Geometry: final body of the model. Coordinates: model frame, mm. Face numbers are marked on the shaded views. A direction names the side the tool comes from. Give positions to 0.01 mm unless a question says otherwise; leave off trailing zeros. Write each loop counter-clockwise with the first axis right and the second up, starting at its lowest first coordinate (ties: lowest second). Pieces come first, ordered by that corner, then holes. Notation, with made-up numbers: M -30,79 L -2,79 A15 cw -2,96 Z; hole C 11,38 d3. An arc over 180 degrees is marked long. Answer as a JSON object with one key per item and string values.
Autodesk Inventor part; units mm, degrees
ref_plane "YZ Plane" through (0, 0, 0) normal (1, 0, 0) x (0, 1, 0)
ref_plane "XZ Plane" through (0, 0, 0) normal (0, 1, 0) x (-1, 0, 0)
ref_plane "XY Plane" through (0, 0, 0) normal (0, 0, 1) x (1, 0, 0)
sketch "スケッチ1" plane through (0, 0, 0) normal (0, 0, 1) x (1, 0, 0)
  line L0 (40.6372, 0) -> (-44.8968, 0)
  line L1 (0, -28.7297) -> (0, 26.7749)
  line L2 (17.5, -15) -> (-17.5, -15)
  line L3 (-17.5, -15) -> (-17.5, 15)
  line L4 (-17.5, 15) -> (17.5, 15)
  line L5 (17.5, 15) -> (17.5, -15)
  point P0 (0, 0)
  dimension "d0" = 35
  dimension "d1" = 30
extrude "押し出し1" add sketch "スケッチ1" along normal blind 30
sketch "スケッチ4" plane through (17.5, -15, 0) normal (1, 0, 0) x (0, 0, -1)
  line L0 (0, 30) -> (0, 0)
  line L1 (0, 30) -> (-30, 30)
  line L2 (-30, 0) -> (-30, 30)
  line L3 (0, 0) -> (-30, 0)
  line L4 (-30, 15) -> (0, 15)
  line L5 (0, 30) -> (-30, 30)
  line L6 (-15, 30) -> (-15, 0)
  circle A0 centre (-15, 15) radius 5
  dimension "d4" = 10
extrude "押し出し2" cut sketch "スケッチ4" against normal through all contours A0 L6 L4 | L4 L6 A0 | L6 L4 A0 | L6 A0 L4
sketch "スケッチ5" plane through (0, 0, 30) normal (0, 0, 1) x (1, 0, 0)
  line L0 (-5.9, -2.4) -> (-5.9, 2.4)
  line L1 (-2.4, -2.4) -> (-5.9, -2.4)
  line L2 (-2.4, -9) -> (-2.4, -2.4)
  line L3 (2.4, -9) -> (-2.4, -9)
  line L4 (2.4, -2.4) -> (2.4, -9)
  line L5 (5.9, -2.4) -> (2.4, -2.4)
  line L6 (5.9, 2.4) -> (5.9, -2.4)
  line L7 (2.4, 2.4) -> (5.9, 2.4)
  line L8 (2.4, 9) -> (2.4, 2.4)
  line L9 (-2.4, 9) -> (2.4, 9)
  line L10 (-2.4, 2.4) -> (-2.4, 9)
  line L11 (-5.9, 2.4) -> (-2.4, 2.4)
  ellipse E0 centre (0.5, 0) end of major axis (4.0355, 0) minor radius 2.5 (0, -2.4749) -> (0, 2.4749) ccw
  ellipse E1 centre (-0.5, 0) end of major axis (-4.0355, 0) minor radius 2.5 (0, 2.4749) -> (0, -2.4749) ccw
  line L12 (-2.6, 9.2) -> (2.6, 9.2)
  line L13 (2.6, 9.2) -> (2.6, 2.6)
  line L14 (2.6, 2.6) -> (6.1, 2.6)
  line L15 (6.1, 2.6) -> (6.1, -2.6)
  line L16 (6.1, -2.6) -> (2.6, -2.6)
  line L17 (2.6, -2.6) -> (2.6, -9.2)
  line L18 (2.6, -9.2) -> (-2.6, -9.2)
  line L19 (-2.6, -9.2) -> (-2.6, -2.6)
  line L20 (-2.6, -2.6) -> (-6.1, -2.6)
  line L21 (-6.1, -2.6) -> (-6.1, 2.6)
  line L22 (-6.1, 2.6) -> (-2.6, 2.6)
  line L23 (-2.6, 2.6) -> (-2.6, 9.2)
  point P0 (0, 0)
  dimension "d9" = 0.2
extrude "押し出し3" cut sketch "スケッチ5" against normal up to surface (30 mm away) contours L0 L11 L10 L9 L8 L7 L6 L5 L4 L3 L2 L1 | E1 E0 | L12 L13 L14 L15 L16 L17 L18 L19 L20 L21 L22 L23
sketch "スケッチ6" plane through (-17.5, 15, 0) normal (0, 1, 0) x (1, 0, 0)
  line L0 (0, 0) -> (35, 0)
  line L1 (0, 0) -> (0, -30)
  line L2 (35, -30) -> (0, -30)
  line L3 (35, 0) -> (35, -30)
  line L4 (35, -10) -> (35, -20)
  line L5 (35, -15) -> (0, -15)
  line L6 (0, -30) -> (35, -30)
  line L7 (17.5, -30) -> (17.5, 0)
  circle A0 centre (7.5246, -15) radius 4.5427
  line L8 (21.5, -7.2467) -> (17.5, -6.2467) construction
  line L9 (17.5, -6.2467) -> (13.5, -7.2467) construction
  spline S0 degree 2 poles (21.5, -7.2467) (17.5, -6.2467) (13.5, -7.2467) knots 1 1 1 2 2 2
  line L10 (21.5, -7.2467) -> (21.5, -5.2467)
  line L11 (21.5, -5.2467) -> (17.5, -2.1432) construction
  line L12 (17.5, -2.1432) -> (13.5, -5.2467) construction
  spline S1 degree 2 poles (21.5, -5.2467) (17.5, -2.1432) (13.5, -5.2467) knots 1 1 1 2 2 2
  line L13 (13.5, -5.2467) -> (13.5, -7.2467)
  circle A1 centre (27.4754, -15) radius 4.5427
  line L14 (13.5, -7.2467) -> (29.7216, -7.2467)
  line L15 (13.5, -5.2467) -> (30.3964, -5.2467)
  dimension "d12" = 2
  dimension "d13" = 4
  dimension "d14" = 4
extrude "顔" add sketch "スケッチ6" along normal blind 2 contours S1 L15 L7 | L7 L15 S1 | A0 L5 | L5 A0 | L15 L10 S0 L7 | L7 S0 L13 L15 | A1 L5 | L5 A1
equation "\"d14\" = d13"
properties part number "head"
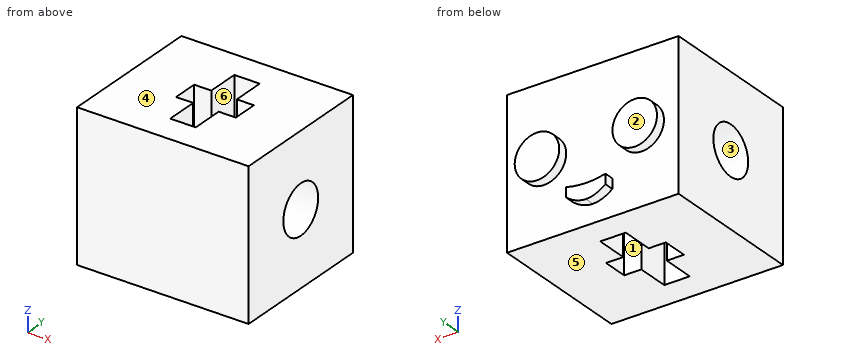
1) Cut plane C-C on z = 15. Return loops of the section in (x, y), and give its area (3 significant figures).
Geometry check:
{"outline": "M -17.5,-15 L 17.5,-15 L 17.5,-5 L 2.6,-5 L 2.6,-9.2 L -2.6,-9.2 L -2.6,-5 L -17.5,-5 Z; M -17.5,5 L -2.6,5 L -2.6,9.2 L 2.6,9.2 L 2.6,5 L 17.5,5 L 17.5,15 L 14.52,15 L 14.52,17 L 5.43,17 L 5.43,15 L -5.43,15 L -5.43,17 L -14.52,17 L -14.52,15 L -17.5,15 Z", "area": "693 mm2"}
2) Cut plane B-B on y = 6. Return loops of the section in (x, z), and give its area (3 significant figures).
Geometry check:
{"outline": "M -17.5,0 L -2.6,0 L -2.6,30 L -17.5,30 Z; M 2.6,0 L 17.5,0 L 17.5,30 L 2.6,30 Z", "area": "894 mm2"}
3) Line query: line 1 (Y direction, x = -4, z = 2); line 2 (X direction, y = 7, z = 2); line 3 (Y direction, x = -13, z = 15). Output: solid intervals per line, ascending. Write a range as from..to.
Geometry check:
{"line 1": "y = -15..-2.6, 2.6..15", "line 2": "x = -17.5..-2.6, 2.6..17.5", "line 3": "y = -15..-5, 5..17"}
4) Contact query for flat-ended pins moving along their axis: P1, Ø1.8, axis at x = 5, z = 8, coming from the +Y side; P2, Ø2, axis at y = 16.5, z = 6, coming from the -X side. Output: stop coordinate, or through.
Geometry check:
{"P1": "stops at y = 15", "P2": "stops at x = -4"}
5) Pull-direction query (Z, two-part tool) for the marked faces 3, 4, 5 and 6; classes: pulls with the +Z half, pulls with the -Z half, needs draft (parallel to the pull), parting line crosses it, or undercut.
Geometry check:
{"face 3": "undercut", "face 4": "pulls with the +Z half", "face 5": "pulls with the -Z half", "face 6": "needs draft"}
6) Cut plane D-D on y = 0. Return loops of the section in (x, z).
Geometry check:
{"outline": "M -17.5,0 L -6.1,0 L -6.1,10 L -17.5,10 Z; M -17.5,20 L -6.1,20 L -6.1,30 L -17.5,30 Z; M 6.1,0 L 17.5,0 L 17.5,10 L 6.1,10 Z; M 6.1,20 L 17.5,20 L 17.5,30 L 6.1,30 Z"}
7) Set-up query: the marked faces 1 and 2. Return all of +Z, -Z, +X, -X, +Y, -Y with unobstructed straight access to the full face (end or side cutting, diameter ignored); none if empty.
Geometry check:
{"face 1": "+Z, -Z", "face 2": "+Z, -Z, +X, -X, +Y"}
8) Cut plane A-A on x = 4.5. Return loops of the section in (y, z), and give its area (3 significant figures).
Geometry check:
{"outline": "M -15,0 L -2.6,0 L -2.6,10.73 A5 cw -2.6,19.27 L -2.6,30 L -15,30 Z; M 2.6,0 L 15,0 L 15,30 L 2.6,30 L 2.6,19.27 A5 cw 2.6,10.73 Z", "area": "715 mm2"}
